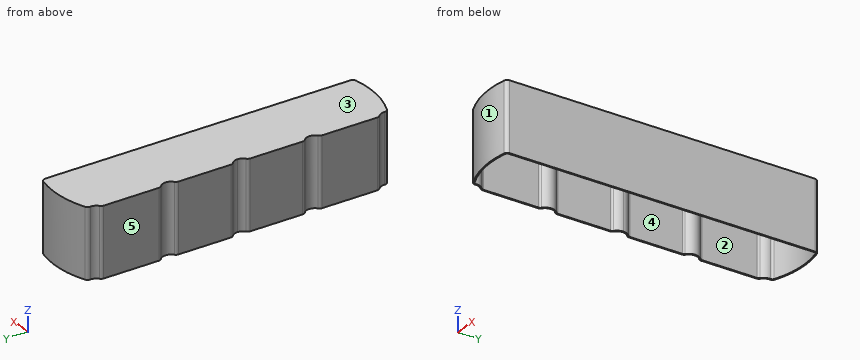
```python
from build123d import *

# Parameters (mm, degrees)
F1_DEPTH = 114.3
F2_T     = -2.032


# Not quite as in the source:
# - ends of sketch curves that miss each other by under 0.0002 mm in the source are joined


with BuildPart() as f1:
    # F0 (on Top) → F1 (new body)
    with BuildSketch(Plane.XY):
        with BuildLine():
            ThreePointArc((-56.5356683944, -224.3892894538), (-55.638228484, -228.1244435583), (-52.7512582129, -230.658645056))
            ThreePointArc((-52.7512582129, -230.658645056), (-8.2827450913, -242.2571362771), (37.5884612507, -239.4631988056))
            ThreePointArc((37.5884612507, -239.4631988056), (41.1635822204, -237.2376139869), (42.5600166876, -233.2646190823))
            Line((42.5600166876, -233.2646190823), (42.5600166876, 15.9969440547))
            Line((42.5600166876, 15.9969440547), (42.5600166876, 16.0075028557))
            Line((42.5600166876, 16.0075028557), (42.5600166876, 265.2690659926))
            ThreePointArc((42.5600166876, 265.2690659926), (41.1635822204, 269.2420608973), (37.5884612507, 271.467645716))
            ThreePointArc((37.5884612507, 271.467645716), (-8.2827450913, 274.2615831875), (-52.7512582129, 262.6630919663))
            ThreePointArc((-52.7512582129, 262.6630919663), (-55.638228484, 260.1288904686), (-56.5356683944, 256.3937363641))
            ThreePointArc((-56.5356683944, 256.3937363641), (-57.6694537634, 249.8005581937), (-61.7387333124, 244.4905269695))
            ThreePointArc((-61.7387333124, 244.4905269695), (-63.4937959622, 242.2831904653), (-64.1199833124, 239.5335598083))
            Line((-64.1199833124, 239.5335598083), (-64.1199833124, 149.3381496402))
            ThreePointArc((-64.1199833124, 149.3381496402), (-63.4937959622, 146.5885189832), (-61.7387333124, 144.3811824789))
            ThreePointArc((-61.7387333124, 144.3811824789), (-56.4999833124, 133.4758547242), (-61.7387333124, 122.5705269695))
            ThreePointArc((-61.7387333124, 122.5705269695), (-63.4937959622, 120.3631904653), (-64.1199833124, 117.6135598083))
            Line((-64.1199833124, 117.6135598083), (-64.1199833124, 31.8632195798))
            ThreePointArc((-64.1199833124, 31.8632195798), (-63.4937959622, 29.1135889227), (-61.7387333124, 26.9062524185))
            ThreePointArc((-61.7387333124, 26.9062524185), (-57.8871404165, 22.0699414424), (-56.5000526478, 16.044938603))
            ThreePointArc((-56.5000526478, 16.044938603), (-56.4999833728, 16.0022234616), (-56.5000526478, 15.9595083074))
            ThreePointArc((-56.5000526478, 15.9595083074), (-57.8871404165, 9.9345054679), (-61.7387333124, 5.0981944918))
            ThreePointArc((-61.7387333124, 5.0981944918), (-63.4937959622, 2.8908579876), (-64.1199833124, 0.1412273306))
            Line((-64.1199833124, 0.1412273306), (-64.1199833124, -85.609112898))
            ThreePointArc((-64.1199833124, -85.609112898), (-63.4937959622, -88.358743555), (-61.7387333124, -90.5660800592))
            ThreePointArc((-61.7387333124, -90.5660800592), (-56.4999833124, -101.4714078139), (-61.7387333124, -112.3767355686))
            ThreePointArc((-61.7387333124, -112.3767355686), (-63.4937959622, -114.5840720728), (-64.1199833124, -117.3337027298))
            Line((-64.1199833124, -117.3337027298), (-64.1199833124, -207.529112898))
            ThreePointArc((-64.1199833124, -207.529112898), (-63.4937959622, -210.278743555), (-61.7387333124, -212.4860800592))
            ThreePointArc((-61.7387333124, -212.4860800592), (-57.6694537634, -217.7961112834), (-56.5356683944, -224.3892894538))
        make_face()
    extrude(amount=F1_DEPTH)

    # F2
    f2_openings = [f1.faces().sort_by_distance(p)[0] for p in [
        (-9.762898, 16.002223, 0),
    ]]
    offset(amount=F2_T, openings=f2_openings, kind=Kind.INTERSECTION)


solid = f1.part
```
Here's how the part is built. I have some questions about the finished solid (model axes, mm). Face numbers are marked on the shaded views. A direction names the side the tool comes from. Coordinates: 2 decimals unless noted, no trailing zeros. Loops run counter-clockwise (first coordinate to the right, second up) from the corner with the lowest first, then second, coordinate; pieces in that order, holes last. Notation, with made-up numbers: M 85,-16.5 L 109,-16.5 A16 cw 109,7.5 Z; hole C -38,46 d7. An arc over 180 degrees is marked long. One line per item, written item: value.
1. Imagine slicing it at A-A (y = -6.5). List the corners of the cut face in (x, z) for me, and give its area (3 significant figures).
Geometry says:
outline: M -64.12,0 L -62.09,0 L -62.09,112.27 L 40.53,112.27 L 40.53,0 L 42.56,0 L 42.56,114.3 L -64.12,114.3 Z
area: 673 mm2
2. Please list where these lines run through material, in increasing order: probe 1 along X at (y, z) = (-208, 107.5); probe 2 along X at (y, z) = (16.5, 69); probe 3 along Z at (x, y) = (0.5, -215).
Geometry says:
probe 1: x = -64.1 to -62.06, 40.53 to 42.56
probe 2: x = -56.51 to -54.48, 40.53 to 42.56
probe 3: z = 112.27 to 114.3
3. Will these pins go through, and if not, where does the flat tip stop? pin 1 Ø8 at (x, z) = (-25.5, 85.5) entering from +Y; pin 2 Ø3 at (x, y) = (-21.5, 103.5) entering from -Z; pin 3 Ø4 at (x, z) = (22.5, 92.5) entering from +Y.
Geometry says:
pin 1: stops at y = 272.36
pin 2: stops at z = 112.27
pin 3: stops at y = 274.22
4. Thinking about a two-plate mould opening in X: for the marked faces 1, 2 and 3, which applies, +X half, -X half, draft (parallel to the pull), parting line (faces both ways), or undercut?
Geometry says:
face 1: parting line
face 2: undercut
face 3: draft
5. On a 3-axis mill with a long thin cutter (end or side, diameter ignored), from which of +Z, -Z, +X, -X, +Y, -Y can I reach the whole of each face in a straight line? I mean the marked faces 4 and 5. Say none if no direction works.
Geometry says:
face 4: -Z
face 5: +Z, -Z, -X, +Y, -Y
6. Imagine slicing it at B-B (x = 4.5). List the corners of the cut face in (y, z) for me.
Geometry says:
outline: M -242.94,0 L -240.91,0 L -240.91,112.27 L 272.91,112.27 L 272.91,0 L 274.94,0 L 274.94,114.3 L -242.94,114.3 Z
